Part model, mm, in its own coordinate system. Round coordinates to 2 decimals unless told otherwise and drop trailing zeros. Loops run counter-clockwise (first coordinate to the right, second up) from the corner with the lowest first, then second, coordinate; pieces in that order, holes last.
from build123d import *

# Parameters (mm, degrees)
CROQUIS1_W              = 440
CROQUIS1_H              = 230
SALIENTE_EXTRUIR1_DEPTH = 3
CROQUIS2_R              = 3.1
CORTAR_EXTRUIR1_DEPTH   = 4
CROQUIS3_W              = 210
CROQUIS3_H              = 130
CORTAR_EXTRUIR2_DEPTH   = 4
CROQUIS4_R              = 11.1
CORTAR_EXTRUIR3_DEPTH   = 4


with BuildPart() as part:
    # Croquis1 → Saliente-Extruir1 (new body)
    with BuildSketch(Plane.XY):
        Rectangle(CROQUIS1_W, CROQUIS1_H)
    extrude(amount=SALIENTE_EXTRUIR1_DEPTH)

    # Croquis2 → Cortar-Extruir1 (cut, through all)
    with BuildSketch(Plane.XY.offset(3)):
        with Locations((-205, 55)):
            Circle(CROQUIS2_R)
        with Locations((-152.5, 100)):
            Circle(CROQUIS2_R)
        with Locations((152.5, 100)):
            Circle(CROQUIS2_R)
        with Locations((-205, -55)):
            Circle(CROQUIS2_R)
        with Locations((205, -55)):
            Circle(CROQUIS2_R)
        with Locations((205, 55)):
            Circle(CROQUIS2_R)
        with Locations((152.5, -100)):
            Circle(CROQUIS2_R)
        with Locations((-152.5, -100)):
            Circle(CROQUIS2_R)
    extrude(amount=-CORTAR_EXTRUIR1_DEPTH, mode=Mode.SUBTRACT)

    # Croquis3 → Cortar-Extruir2 (cut, through all)
    with BuildSketch(Plane(origin=(0, 0, 0), x_dir=(-1, 0, 0), z_dir=(0, 0, -1))):
        with Locations((0, -20)):
            Rectangle(CROQUIS3_W, CROQUIS3_H)
    extrude(amount=-CORTAR_EXTRUIR2_DEPTH, mode=Mode.SUBTRACT)

    # Croquis4 → Cortar-Extruir3 (cut, through all)
    with BuildSketch(Plane(origin=(0, 0, 0), x_dir=(-1, 0, 0), z_dir=(0, 0, -1))):
        with Locations((-40, 80)):
            Circle(CROQUIS4_R)
    extrude(amount=-CORTAR_EXTRUIR3_DEPTH, mode=Mode.SUBTRACT)


solid = part.part
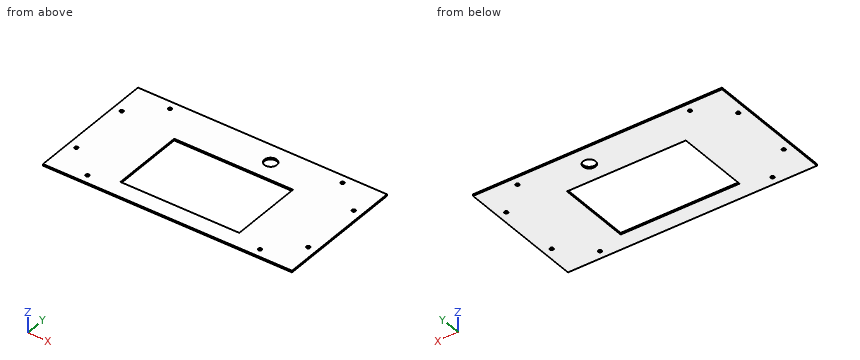
1) Slice it at C-C, the plane z = 1.05. Give the number of separate pieces and of enclosed holes in the cut face, then the cut area to 3 significant figures.
Values:
separate pieces: 1
enclosed holes: 10
area: 73,300 mm2
2) Drop a flat-ended pin along its axis: pin 1 Ø3.5 at (x, y) = (-205, 55) entering from -Z. Give the stop position or say it passes through.
Values:
pin 1: passes through
3) Slice it at D-D, the plane x = -71. Give the cut face in (y, z), then the cut area to 3 significant figures.
Values:
outline: (-115, 0) - (-85, 0) - (-85, 3) - (-115, 3) - close; (45, 0) - (115, 0) - (115, 3) - (45, 3) - close
area: 300 mm2
4) Slice it at B-B, the plane x = 40. Give the cut face in (y, z), then the cut area to 3 significant figures.
Values:
outline: (-115, 0) - (-85, 0) - (-85, 3) - (-115, 3) - close; (45, 0) - (68.9, 0) - (68.9, 3) - (45, 3) - close; (91.1, 0) - (115, 0) - (115, 3) - (91.1, 3) - close
area: 233 mm2
5) Wall check: line 1 along Y through (x, z) = (152.5, 1.95); line 2 along Y through (x, z) = (40, 0.8); line 3 along Y through (x, z) = (-17, 0.1). Give the ranges that are in metal, low to high.
Values:
line 1: y = -115 to -103.1, -96.9 to 96.9, 103.1 to 115
line 2: y = -115 to -85, 45 to 68.9, 91.1 to 115
line 3: y = -115 to -85, 45 to 115
6) Slice it at A-A, the plane y = 80. Give the cut face in (x, z).
Values:
outline: (-220, 0) - (28.9, 0) - (28.9, 3) - (-220, 3) - close; (51.1, 0) - (220, 0) - (220, 3) - (51.1, 3) - close
